Geometry check sheet. Reference: the model listing, model coordinates, mm. A direction names the side the tool comes from. Coordinates: 2 decimals unless noted, no trailing zeros. Write each loop counter-clockwise with the first axis right and the second up, starting at its lowest first coordinate (ties: lowest second). Pieces come first, ordered by that corner, then holes. Notation, with made-up numbers: (15.5, -39.5) -> (73.5, -39.5) arc R3 cw to (73.5, -34.5) -> close; hole circle Ø4 at (28.5, -14). An arc over 180 degrees is marked (long way). Answer as CSV lines item,"result".
```python
from build123d import *

# Parameters (mm, degrees)
BOSS_EXTRUDE1_DEPTH     = 8.5
CUT_EXTRUDE1_DEPTH      = 24.334523779
CUT_EXTRUDE1_DEPTH_BACK = 2.5
SKETCH2_W               = 16
SKETCH2_H               = 14
SKETCH3_W               = 3
SKETCH3_H               = 3
SKETCH3_R               = 0.6
BOSS_EXTRUDE2_DEPTH     = 1
BOSS_EXTRUDE3_DEPTH     = 18.5
SKETCH5_R               = 5
BOSS_EXTRUDE4_DEPTH     = 6
CUT_EXTRUDE2_START      = -3
CUT_EXTRUDE2_DEPTH      = 3
SKETCH7_R               = 1
SKETCH7_R_2             = 0.7
BOSS_EXTRUDE5_DEPTH     = 4.5


with BuildPart() as part:
    # Sketch1 → Boss-Extrude1 (new, symmetric)
    with BuildSketch(Plane.XY):
        with BuildLine():
            Line((-8.5, 5), (-8.5, -5))
            Line((-8.5, -5), (8.5, -5))
            Line((8.5, -5), (8.5, 5))
            Line((8.5, 5), (3.5, 5))
            Line((3.5, 5), (3.5, 16))
            Line((3.5, 16), (1, 16))
            ThreePointArc((1, 16), (0, 17), (1, 18))
            Line((1, 18), (3.5, 18))
            Line((3.5, 18), (3.5, 19))
            Line((3.5, 19), (8.5, 19))
            Line((8.5, 19), (8.5, 20))
            Line((8.5, 20), (-3.5, 20))
            Line((-3.5, 20), (-3.5, 5))
            Line((-3.5, 5), (-8.5, 5))
        make_face()
    extrude(amount=BOSS_EXTRUDE1_DEPTH, both=True)

    # Sketch2 → Cut-Extrude1 (cut, two sides: drawn at the far end of the back side and taken through both)
    with BuildSketch(Plane(origin=(0, 0, 0), x_dir=(0, 0, -1), z_dir=(1, 0, 0)).offset(-CUT_EXTRUDE1_DEPTH_BACK)):
        with Locations((0.5, 12)):
            Rectangle(SKETCH2_W, SKETCH2_H)
    extrude(amount=CUT_EXTRUDE1_DEPTH + CUT_EXTRUDE1_DEPTH_BACK, mode=Mode.SUBTRACT)

    # Sketch3 → Boss-Extrude2 (add)
    with BuildSketch(Plane(origin=(0, 0, -8.5), x_dir=(-1, 0, 0), z_dir=(0, 0, -1))):
        with Locations((1, 6.5)):
            Rectangle(SKETCH3_W, SKETCH3_H)
        with Locations((1, 6.5)):
            Circle(SKETCH3_R, mode=Mode.SUBTRACT)
    extrude(amount=-BOSS_EXTRUDE2_DEPTH)

    # Sketch4 → Boss-Extrude3 (add)
    with BuildSketch(Plane.ZY.offset(3.5)):
        with BuildLine():
            Line((-5.562148865, 18.25), (5.562148865, 18.25))
            ThreePointArc((5.562148865, 18.25), (8, 12.5), (5.562148865, 6.75))
            Line((5.562148865, 6.75), (-5.562148865, 6.75))
            ThreePointArc((-5.562148865, 6.75), (-8, 12.5), (-5.562148865, 18.25))
        make_face()
    extrude(amount=BOSS_EXTRUDE3_DEPTH)

    # Sketch5 → Boss-Extrude4 (add)
    with BuildSketch(Plane(origin=(-2.5, 0, 0), x_dir=(0, 0, -1), z_dir=(1, 0, 0))):
        with Locations(Location((0, 12.5, 0), (0, 0, 90))):
            Circle(SKETCH5_R)
    extrude(amount=BOSS_EXTRUDE4_DEPTH)

    # Sketch6 → Cut-Extrude2 (cut)
    with BuildSketch(Plane(origin=(3.5, 0, 0), x_dir=(0, 0, -1), z_dir=(1, 0, 0)).offset(CUT_EXTRUDE2_START)):
        with BuildLine():
            Line((4.111517555, 15.345245752), (2.055758778, 13.922622876))
            ThreePointArc((2.055758778, 13.922622876), (-1.422622876, 14.555758778), (-2.055758778, 11.077377124))
            Line((-2.055758778, 11.077377124), (-4.111517555, 9.654754248))
            ThreePointArc((-4.111517555, 9.654754248), (-2.845245752, 16.611517555), (4.111517555, 15.345245752))
        make_face()
    extrude(amount=CUT_EXTRUDE2_DEPTH, mode=Mode.SUBTRACT)

    # Sketch7 → Boss-Extrude5 (add)
    # profile 1 of 2: a face of its own
    with BuildSketch(Plane.ZY.offset(8.5)):
        with Locations(Location((-3.75, -2.301826995, 0), (0, 0, 180))):
            Circle(SKETCH7_R)
        with Locations((-3.75, -2.301826995)):
            Circle(SKETCH7_R_2, mode=Mode.SUBTRACT)
    # profile 2 of 2: a face of its own
    with BuildSketch(Plane.ZY.offset(8.5)):
        with Locations(Location((3.75, -2.301826995, 0), (0, 0, 180))):
            Circle(SKETCH7_R)
        with Locations((3.75, -2.301826995)):
            Circle(SKETCH7_R_2, mode=Mode.SUBTRACT)
    extrude(amount=BOSS_EXTRUDE5_DEPTH)


solid = part.part
```
Item 1: Cross-section at D-D, the plane y = 12.5. Record the cut outline in (x, z).
Responses:
outline,"(-22, -8) -> (-3.5, -8) -> (-3.5, -8.5) -> (-2.5, -8.5) -> (-2.5, -5) -> (3.5, -5) -> (3.5, 2.5) -> (0.5, 2.5) -> (0.5, 5) -> (-2.5, 5) -> (-2.5, 7.5) -> (3.5, 7.5) -> (3.5, 8.5) -> (-3.5, 8.5) -> (-3.5, 8) -> (-22, 8) -> close"
Item 2: Depth check by flat-ended pin: pin 1 Ø5 at (x, y) = (-16, 7.5) entering from +Z; pin 2 Ø8.5 at (y, z) = (13.5, -1) entering from +X; pin 3 Ø1 at (y, z) = (8, -5) entering from +X. Enter the tip coordinate at first touch or a pass-through.
Responses:
pin 1,"stops at z = 7.6"
pin 2,"stops at x = 3.5"
pin 3,"stops at x = -2.5"
Item 3: Release check for a two-part mould opening along Z. For faces 6 (the flat face through (3, 5, 0)), 7 (the cylindrical face through (-10.72, -2.27, 3.05)), 8 (the flat face through (0, 2, -8.5)), 9 (the cylindrical face through (0, 17, 8)) record: +Z half, -Z half, draft (parallel to the pull), parting line (faces both ways), or undercut.
Responses:
face 6,"undercut"
face 7,"undercut"
face 8,"-Z half"
face 9,"draft"
Item 4: Cross-section at C-C, the plane z = 0. Record the cut outline in (x, y), plus the area to 3 significant figures.
Responses:
outline,"(-22, 6.75) -> (-3.5, 6.75) -> (-3.5, 5) -> (-8.5, 5) -> (-8.5, -5) -> (8.5, -5) -> (8.5, 5) -> (-2.5, 5) -> (-2.5, 7.5) -> (3.5, 7.5) -> (3.5, 15) -> (0.5, 15) -> (0.5, 17.5) -> (-2.5, 17.5) -> (-2.5, 19) -> (8.5, 19) -> (8.5, 20) -> (-3.5, 20) -> (-3.5, 18.25) -> (-22, 18.25) -> close"
area,"461 mm2"
Item 5: Cross-section at B-B, the plane x = 4.5. Record the cut outline in (y, z), plus the area to 3 significant figures.
Responses:
outline,"(-5, -8.5) -> (5, -8.5) -> (5, 8.5) -> (-5, 8.5) -> close; (19, -8.5) -> (20, -8.5) -> (20, 8.5) -> (19, 8.5) -> close"
area,"187 mm2"
Item 6: Thickness scan on probe 1 along Y at (x, z) = (-1, -8.2); probe 2 along Y at (x, z) = (-9.9, -3.75); probe 3 along Y at (x, z) = (5.5, -1). Record the ranges inside material, lowest first.
Responses:
probe 1,"y = -5 to 5.9, 7.1 to 8, 19 to 20"
probe 2,"y = -3.3 to -3, -1.6 to -1.3, 6.75 to 18.25"
probe 3,"y = -5 to 5, 19 to 20"
Item 7: Set-up check for faces 1 (the flat face through (-8.5, -2, 4)), 2 (the flat face through (0, 7, -7.5)), 3 (the flat face through (3.5, 11, 0)), 4 (the flat face through (8.5, 0, 0)), 5 (the flat face through (0.5, 6, -8)): record each of +Z, -Z, +X, -X, +Y, -Y from which the full face is reachable in a straight line by a thin tool's end or side.
Responses:
face 1,"-X"
face 2,"+X"
face 3,"+Z, -Z, +X"
face 4,"+Z, -Z, +X, +Y, -Y"
face 5,"-Z, +X"
Item 8: Cross-section at A-A, the plane x = -1. Record the cut outline in (y, z), plus the area to 3 significant figures.
Responses:
outline,"(-5, -8.5) -> (5.9, -8.5) -> (5.9, -7.5) -> (5, -7.5) -> (5, 7.5) -> (19, 7.5) -> (19, -8.5) -> (20, -8.5) -> (20, 8.5) -> (-5, 8.5) -> close; (7.1, -8.5) -> (8, -8.5) -> (8, -7.5) -> (7.1, -7.5) -> close; circle Ø10 at (12.5, 0)"
area,"281 mm2"
